```python
from build123d import *

# Parameters (mm, degrees)
SKETCH2_R            = 67.5
BOSS_EXTRUDE2_DEPTH  = 11
SKETCH3_R            = 66
CUT_EXTRUDE11_DEPTH  = 3
BOSS_EXTRUDE3_DEPTH  = 63.34
BOSS_EXTRUDE10_DEPTH = 12.25
BOSS_EXTRUDE11_DEPTH = 12.25
BOSS_EXTRUDE12_START = -12.25
BOSS_EXTRUDE12_DEPTH = 4.25
BOSS_EXTRUDE13_DEPTH = 12.25
SKETCH4_10_R         = 2.5273
CUT_EXTRUDE12_DEPTH  = 12.25


# Read off the part's stored shape, not the designer's step: Boss-Extrude12
with BuildPart() as part:
    # Sketch2 → Boss-Extrude2 (new body)
    with BuildSketch(Plane.XY):
        Circle(SKETCH2_R)
    extrude(amount=BOSS_EXTRUDE2_DEPTH)

    # Sketch3 → Cut-Extrude11 (cut)
    with BuildSketch(Plane(origin=(0, 0, 0), x_dir=(-1, 0, 0), z_dir=(0, 0, -1))):
        Circle(SKETCH3_R)
    extrude(amount=-CUT_EXTRUDE11_DEPTH, mode=Mode.SUBTRACT)

    # Sketch4 → Boss-Extrude3 (add)
    with BuildSketch(Plane(origin=(0, 0, 3), x_dir=(-1, 0, 0), z_dir=(0, 0, -1))):
        Polygon((-36.106368438, -18.003584956), (-28.133944044, -17.408739697), (-28.729209741, -9.430900362), (-36.701616568, -10.025761076), (-36.627210549, -11.022989106), align=None)
        Polygon((2.114943846, -43.743465349), (10.09276687, -43.148200869), (9.49750239, -35.170377845), (1.519679366, -35.765642325), align=None)
        Polygon((31.67620014, 10.293427606), (31.75060616, 9.296199576), (23.772783163, 8.700934735), (23.177535005, 16.678758977), (31.155358029, 17.274023457), align=None)
        Polygon((-7.664290982, 42.969259013), (-15.642114006, 42.373994533), (-15.046849526, 34.396171509), (-7.069026502, 34.991435989), align=None)
    extrude(amount=-BOSS_EXTRUDE3_DEPTH)



with BuildPart() as body_2:
    # Sketch4<6> → Boss-Extrude10 (new body)
    with BuildSketch(Plane(origin=(0, 0, 3), x_dir=(-1, 0, 0), z_dir=(0, 0, -1))):
        Polygon((-37.237933985, 29.544025614), (-53.20294076, 28.352798205), (-50.189331626, -12.034925436), (-36.627210549, -11.022989106), (-36.701616568, -10.025761076), (-49.266513848, -10.96328965), (-52.131302781, 27.429978539), (-37.163525925, 28.546797736), align=None)
    extrude(amount=-BOSS_EXTRUDE10_DEPTH)


with BuildPart() as part_1:
    add(part.part)

    add(body_2.part)  # Boss-Extrude11 merges body 2
    # Sketch4<7> → Boss-Extrude11 (add)
    with BuildSketch(Plane(origin=(0, 0, 3), x_dir=(-1, 0, 0), z_dir=(0, 0, -1))):
        Polygon((-15.463534662, 39.980647626), (-15.537942722, 40.977875504), (-39.960658599, 39.155576962), (-39.232389741, 29.395209494), (-38.235161863, 29.469617554), (-38.889022661, 38.232757144), align=None)
        Polygon((6.002179443, 42.585089599), (-7.560119698, 41.573139984), (-7.485711638, 40.575912106), (5.079359625, 41.513453661), (7.61667447, 7.507983023), (8.613902348, 7.582391083), align=None)
    extrude(amount=-BOSS_EXTRUDE11_DEPTH)

    # Boss-Extrude12 outline → Boss-Extrude12 (add)
    with BuildSketch(Plane(origin=(0, 0, 3), x_dir=(-1, 0, 0), z_dir=(0, 0, -1)).offset(BOSS_EXTRUDE12_START)):
        Polygon((31.67620014, 10.293427606), (31.75060616, 9.296199576), (44.714394547, 10.263491961), (47.579183525, -28.129776815), (32.611406667, -29.246596012), (32.685814727, -30.24382389), (33.683042605, -30.16941583), (34.336903403, -38.93255542), (9.914187526, -40.754853962), (9.988595586, -41.75208184), (35.408539341, -39.855375238), (34.680270483, -30.09500777), (48.650821503, -29.05259648), (45.637212368, 11.33512716), align=None)
        Polygon((-13.619910772, -2.199099303), (-30.173893546, -3.434273099), (-30.099485486, -4.431500977), (-13.545502712, -3.196327181), (-10.5542987, -43.284887875), (2.010772562, -42.347346319), (1.936364502, -41.350118441), (-9.631478882, -42.213251937), (-12.771499014, -0.130235487), (-1.826827461, 0.686400104), (-1.901235521, 1.683627982), (-13.843134952, 0.792584331), align=None)
        Polygon((25.621774288, 2.734474823), (25.547366228, 3.731702701), (8.892344879, 2.488989922), (8.966752939, 1.491762044), align=None)
    extrude(amount=BOSS_EXTRUDE12_DEPTH)

    # Sketch4<9> → Boss-Extrude13 (add)
    with BuildSketch(Plane(origin=(0, 0, 3), x_dir=(-1, 0, 0), z_dir=(0, 0, -1))):
        Polygon((-50.748151509, -4.545744855), (-51.343432315, 3.432076951), (-58.324046353, 2.911219122), (-57.728798463, -5.06660514), align=None)
        Polygon((-52.161943422, 14.401581934), (-52.757224228, 22.379403739), (-59.737760091, 21.858551743), (-59.142512201, 13.880727481), align=None)
        Polygon((46.196032252, 3.845946579), (46.791313057, -4.131875227), (53.771927095, -3.611017397), (53.176679206, 4.366806864), align=None)
        Polygon((47.609824165, -15.10138021), (48.205104971, -23.079202015), (55.185640833, -22.558350019), (54.590392944, -14.580525757), align=None)
    extrude(amount=-BOSS_EXTRUDE13_DEPTH)

    # Sketch4<10> → Cut-Extrude12 (cut)
    with BuildSketch(Plane(origin=(0, 0, 3), x_dir=(-1, 0, 0), z_dir=(0, 0, -1))):
        with Locations((-32.5, 50.435602505)):
            Circle(SKETCH4_10_R)
        with Locations((-32.5, -50.435602505)):
            Circle(SKETCH4_10_R)
        with Locations((32.5, -50.435602505)):
            Circle(SKETCH4_10_R)
        with Locations((32.5, 50.435602505)):
            Circle(SKETCH4_10_R)
    extrude(amount=-CUT_EXTRUDE12_DEPTH, mode=Mode.SUBTRACT)


solid = part_1.part
```
For this review, take the finished solid that the model builds, in its own axes (mm). A direction names the side the tool comes from. Round coordinates to 2 decimals unless told otherwise and drop trailing zeros. Write each loop counter-clockwise with the first axis right and the second up, starting at its lowest first coordinate (ties: lowest second). Pieces come first, ordered by that corner, then holes. Notation, with made-up numbers: (25.25, -22.75) -> (77.25, -22.75) arc R16 cw to (77.25, 4.25) -> close; hole circle Ø3 at (-20, 72). An arc over 180 degrees is marked (long way). One line per question, with ' | ' between items. Start each with the question number.
(1) Mouldability with a two-part tool opening along Y and no side actions: class faces 5 (the face through (58.03, -1.02, 13.1)), 6 (the face through (52, 15, 15.25)), 7 (the face through (-49.74, 4.11, 13.1)), 8 (the face through (-33.666, -52.678, 6.944)) as released by +Y, released by -Y, zero draft, split by the parting line, or undercut.
(2) Insertion check: P1, Ø1.1, axis at x = -16, y = 2.5, coming from the +Z side; P2, Ø6, axis at x = -32.5, y = 50.44, coming from the -Z side; P3, Ø3, axis at x = 29, z = 14.5, coming from the +Y side. Each pin has a flat end and moves straight along its axis. Give the tip position at first contact, or say it passes through.
(3) Tool access review of faces 1 (the face through (12.07, -22.96, 13.15)), 2 (the face through (7.376, 0.272, 13.155)), 3 (the face through (1, 1, 3)), 4 (the face through (-54.892, -18.625, 13.095)): name each direction out of +Z, -Z, +X, -X, +Y, -Y from which nothing blocks a thin tool from reaching the whole face with its end or side.
(4) For line 1 along Y through (x, z) = (-32.5, 8.75); line 2 along Y through (x, z) = (-32, 7); line 3 along Z through (x, y) = (-3.5, -31), list the stretches that pass through material, from the lowest coordinate up. Write a range as from..to.
(5) Add section B-B, the plane x = 32.5. Write out the cut boundary in (y, z).
(6) Add section D-D, the plane z = 13.5. Give the number of separate pieces and of enclosed holes in the cut face, plus the area to 3 significant figures.
(7) Add section A-A, the plane z = 38.5. Write out the cut boundary in (x, y), plus the area to 3 significant figures.
(8) Add section C-C, the plane y = -20. Write out the cut boundary in (x, z).
Answer list:
1) face 5: released by -Y | face 6: zero draft | face 7: released by +Y | face 8: undercut
2) P1: z = 15.25 | P2: z = 3 | P3: y = 40.09
3) face 1: +Z, -Y | face 2: +Z | face 3: -Z | face 4: +Z, -X, +Y
4) line 1: -59.16..-52.96, -47.91..47.91, 52.96..59.16 | line 2: -59.43..-52.91, -47.96..47.96, 52.91..59.43 | line 3: 3..11
5) outline: (-59.16, 0) -> (-57.44, 0) -> (-57.44, 3) -> (-52.96, 3) -> (-52.96, 11) -> (-59.16, 11) -> close; (-47.91, 3) -> (47.91, 3) -> (47.91, 11) -> (39.71, 11) -> (39.71, 15.25) -> (38.71, 15.25) -> (38.71, 11) -> (-9.71, 11) -> (-9.71, 66.34) -> (-17.73, 66.34) -> (-17.73, 11) -> (-47.91, 11) -> close; (52.96, 3) -> (57.44, 3) -> (57.44, 0) -> (59.16, 0) -> (59.16, 11) -> (52.96, 11) -> close
6) separate pieces: 3 | enclosed holes: 0 | area: 832 mm²
7) outline: (-31.75, 9.3) -> (-23.77, 8.7) -> (-23.18, 16.68) -> (-31.16, 17.27) -> close; (-10.09, -43.15) -> (-2.11, -43.74) -> (-1.52, -35.77) -> (-9.5, -35.17) -> close; (7.07, 34.99) -> (15.05, 34.4) -> (15.64, 42.37) -> (7.66, 42.97) -> close; (28.13, -17.41) -> (36.11, -18) -> (36.7, -10.03) -> (28.73, -9.43) -> close | area: 256 mm²
8) outline: (-64.47, 0) -> (-62.9, 0) -> (-62.9, 3) -> (62.9, 3) -> (62.9, 0) -> (64.47, 0) -> (64.47, 11) -> (12.29, 11) -> (12.29, 15.25) -> (11.29, 15.25) -> (11.29, 11) -> (-46.97, 11) -> (-46.97, 15.25) -> (-54.99, 15.25) -> (-54.99, 11) -> (-64.47, 11) -> close
